The model under review builds one solid part; all positions refer to its coordinate system, in mm. A direction names the side the tool comes from. Coordinates: 2 decimals unless noted, no trailing zeros. Loops run counter-clockwise (first coordinate to the right, second up) from the corner with the lowest first, then second, coordinate; pieces in that order, holes last. Notation, with made-up numbers: (43.25, 81) - (94.25, 81) arc R19 cw to (94.25, 100) - close; hole circle Ø4 at (-13, -16). An arc over 180 degrees is marked (long way). Answer in a Markdown table with one row per item. Add a question column.
(1) Mouldability with a two-part tool opening along Z and no side actions: class faces 3 (the flat face through (326, 21, -41.275)), 4 (the cylindrical face through (238.04, -1.61, -5.273)), 5 (the flat face through (326, -3.175, -18)) as +Z half, -Z half, draft (parallel to the pull), parting line (faces both ways), or undercut.
(2) For line 1 along X through (y, z) = (-2.2, -25.4); line 2 along Z through (x, y) = (398, 15) (3 decimals); line 3 along Y through (x, z) = (631, -27) (3 decimals), list the stretches that pass through material, from the lowest coordinate up.
(3) We need section A-A on x = 241.3. Write out the cut boundary in (y, z) (3 decimals).
(4) Machinability: for faces 1 (the flat face through (326, 20, -38.1)), 2 (the cylindrical face through (263.44, -1.61, -5.273)), which of the approach directions +Z, -Z, +X, -X, +Y, -Y give a long, thin tool a straight path to every point of the face, cutting with its end or side? Answer none if there is none.
(5) For P1, Ø12.5, axis at x = 393.7, z = -9.525, coming from the -Y side (3 decimals); P2, Ø9, axis at x = 15.875, y = 12.7, coming from the +Z side; P3, Ø9, axis at x = 650.875, z = -25.4, coming from the +Y side; P4, Ø1, axis at x = 211, z = -36.5, coming from the -Y side, all flat-tipped, find the tip position at first contact; note any pin that passes through.
from build123d import *

# Parameters (mm, degrees)
BASE_FLANGE1_DEPTH = 660.4
SKETCH3_R          = 3.429
SKETCH3_R_2        = 5.3578125
CUT_EXTRUDE2_DEPTH = 6.35
FILLET1_R          = 3.175
SKETCH4_R          = 3.429
CUT_EXTRUDE3_DEPTH = 3.175


# Sheet-metal steps are written as plain solids
with BuildPart() as part:
    # Sketch1 → Base-Flange1 (new body)
    with BuildSketch(Plane(origin=(0, 0, 0), x_dir=(0, 0, -1), z_dir=(1, 0, 0))):
        with BuildLine():
            Line((0, 0), (34.925, 0))
            ThreePointArc((34.925, 0), (37.17006403, 0.92993597), (38.1, 3.175))
            Line((38.1, 3.175), (38.1, 38.1))
            Line((38.1, 38.1), (41.275, 38.1))
            Line((41.275, 38.1), (41.275, 3.175))
            ThreePointArc((41.275, 3.175), (39.415128061, -1.315128061), (34.925, -3.175))
            Line((34.925, -3.175), (0, -3.175))
            Line((0, -3.175), (0, 0))
        make_face()
    extrude(amount=BASE_FLANGE1_DEPTH)

    # Sketch3 → Cut-Extrude2 (cut)
    with BuildSketch(Plane.XZ.offset(3.175)):
        with Locations(Location((9.525, -25.4, 0), (0, 0, 270))):
            Circle(SKETCH3_R)
        with Locations(Location((9.525, -6.35, 0), (0, 0, 270))):
            Circle(SKETCH3_R)
        with Locations(Location((650.875, -25.4, 0), (0, 0, 270))):
            Circle(SKETCH3_R)
        with Locations(Location((650.875, -6.35, 0), (0, 0, 270))):
            Circle(SKETCH3_R)
        with Locations(Location((241.3, -9.525, 0), (0, 0, 270))):
            Circle(SKETCH3_R_2)
        with Locations(Location((419.1, -9.525, 0), (0, 0, 270))):
            Circle(SKETCH3_R_2)
        with Locations(Location((266.7, -9.525, 0), (0, 0, 270))):
            Circle(SKETCH3_R_2)
        with Locations(Location((393.7, -9.525, 0), (0, 0, 270))):
            Circle(SKETCH3_R_2)
    extrude(amount=-CUT_EXTRUDE2_DEPTH, mode=Mode.SUBTRACT)

    # Fillet1
    fillet1_edges = [part.edges().sort_by_distance(p)[0] for p in [
        (660.4, -1.5875, 0),
        (0, -1.5875, 0),
        (660.4, 38.1, -39.6875),
        (0, 38.1, -39.6875),
    ]]
    fillet(fillet1_edges, radius=FILLET1_R)

    # Sketch4 → Cut-Extrude3 (cut)
    with BuildSketch(Plane(origin=(0, 0, -41.275), x_dir=(-1, 0, 0), z_dir=(0, 0, -1))):
        with Locations((-644.525, 31.75)):
            Circle(SKETCH4_R)
        with Locations((-644.525, 12.7)):
            Circle(SKETCH4_R)
        with Locations((-15.875, 31.75)):
            Circle(SKETCH4_R)
        with Locations((-15.875, 12.7)):
            Circle(SKETCH4_R)
    extrude(amount=-CUT_EXTRUDE3_DEPTH, mode=Mode.SUBTRACT)


solid = part.part
Outcome:
| question | item | result |
|---|---|---|
| 1 | face 3 | -Z half |
| 1 | face 4 | undercut |
| 1 | face 5 | draft |
| 2 | line 1 | 0 to 6.1, 12.95 to 647.45, 654.3 to 660.4 |
| 2 | line 2 | -41.275 to -38.1 |
| 2 | line 3 | -3.175 to 0 |
| 3 | outline | (-3.175, -34.925) arc R6.35 ccw to (3.175, -41.275) - (38.1, -41.275) - (38.1, -38.1) - (3.175, -38.1) arc R3.175 cw to (0, -34.925) - (0, -14.883) - (-3.175, -14.883) - close; (-3.175, -4.167) - (0, -4.167) - (0, 0) - (-3.175, 0) - close |
| 4 | face 1 | +Z, +X, -X, +Y |
| 4 | face 2 | +Y, -Y |
| 5 | P1 | y = -3.175 |
| 5 | P2 | z = -38.1 |
| 5 | P3 | y = 0 |
| 5 | P4 | y = -3.08 |
